Part model, mm, in its own coordinate system. A direction names the side the tool comes from. Coordinates: 2 decimals unless noted, no trailing zeros. Loops run counter-clockwise (first coordinate to the right, second up) from the corner with the lowest first, then second, coordinate; pieces in that order, holes last. Notation, with made-up numbers: (-10.5, -6) - (26.5, -6) arc R11 ccw to (26.5, 5) - close; hole circle Ø11 at (41.25, -13). An arc over 180 degrees is marked (long way). Use a Markdown table: item, result. Add a question column.
1. Wall check: probe 1 along Y at (x, z) = (-70.5, -14.5); probe 2 along X at (y, z) = (-63, -44); probe 3 along X at (y, z) = (-62, 33). Give the ranges that are in metal, low to high. Write a range as [from, to].
2. Pull direction Z, two halves, no side cores. Call faces 3 (the flat face through (-2, 0, 1)), 4 (the cylindrical face through (55.5, -50.3, -41.6)), 5 (the flat face through (-2, -6, 81.1)): pulls with the +Z half, pulls with the -Z half, needs draft (parallel to the pull), parting line crosses it, or undercut.
3. Band-saw the part on B-B, the plane z = 12.5. Give the cut face in (x, y), plus the area to 3 significant figures.
4. Band-saw the part on D-D, the plane x = 16.5. Give the cut face in (y, z), plus the area to 3 significant figures.
5. Drop flat-ended pins along their axis: pin 1 (2 mm diameter, centred on y = -36, z = 26, fed in from -X); pin 2 (5 mm diameter, centred on y = -38.5, z = -37, fed in from +X). Give the stop position or say it passes through.
6. Band-saw the part on A-A, the plane y = -20. Give the cut face in (x, z).
7. 3-axis set-ups, long thin cutter, end or side, ignore diameter. For faces 1 (the flat face through (129.614, -6, -1)), 2 (the cylindrical face through (65.6, -50.27, 22.05)): which of +Z, -Z, +X, -X, +Y, -Y reach the whole face in a straight line?
8. Band-saw the part on C-C, the plane x = 60. Give the cut face in (y, z), plus the area to 3 significant figures.
from build123d import *

# Parameters (mm, degrees)
F0_W     = 259.227424
F0_H     = 162.200198
F1_DEPTH = 12.7
F2_R     = 8.763
F3_DEPTH = 76.2
F4_R     = 6.35
F5_DEPTH = 76.2


with BuildPart() as f1:
    # F0 (on Front) → F1 (new body)
    with BuildSketch(Plane.XZ):
        Rectangle(F0_W, F0_H)
    extrude(amount=F1_DEPTH)

    # F2 (on face) → F3 (join)
    with BuildSketch(Plane.XZ.offset(12.7)):
        with Locations((57.503741, 25.405739)):
            Circle(F2_R)
    extrude(amount=F3_DEPTH)

    # F4 (on face) → F5 (join)
    with BuildSketch(Plane.XZ.offset(12.7)):
        with Locations((49.444617, -43.506545)):
            Circle(F4_R)
    extrude(amount=F5_DEPTH)


solid = f1.part
Geometry check:
| question | item | result |
|---|---|---|
| 1 | probe 1 | y = [-12.7, 0] |
| 1 | probe 2 | x = [43.11, 55.78] |
| 1 | probe 3 | x = [53.13, 61.88] |
| 2 | face 3 | needs draft |
| 2 | face 4 | undercut |
| 2 | face 5 | pulls with the +Z half |
| 3 | outline | (-129.61, -12.7) - (129.61, -12.7) - (129.61, 0) - (-129.61, 0) - close |
| 3 | area | 3,290 mm^2 |
| 4 | outline | (-12.7, -81.1) - (0, -81.1) - (0, 81.1) - (-12.7, 81.1) - close |
| 4 | area | 2,060 mm^2 |
| 5 | pin 1 | stops at x = 48.74 |
| 5 | pin 2 | stops at x = 54.37 |
| 6 | outline | circle Ø12.7 at (49.44, -43.51); circle Ø17.53 at (57.5, 25.41) |
| 7 | face 1 | +Z, -Z, +X, +Y, -Y |
| 7 | face 2 | -Y |
| 8 | outline | (-88.9, 17.01) - (-12.7, 17.01) - (-12.7, -81.1) - (0, -81.1) - (0, 81.1) - (-12.7, 81.1) - (-12.7, 33.81) - (-88.9, 33.81) - close |
| 8 | area | 3,340 mm^2 |
